Study the drawing (mm; zero at the part's minimum x, y, z) and answer. Give positions to 0.01 mm unless a question says otherwise; leave off trailing zeros. Write each loop counter-clockwise with the first axis right and the second up, starting at its lowest first coordinate (ties: lowest second). Pieces come first, ordered by that corner, then holes.
1) Find section A-A (y = 112). Determine the outline of the cut face in (x, z), plus the area to 3 significant figures.
2) Given pin 1 Ø3 at (y, z) = (112, 5) entering from -X; pin 2 Ø8 at (y, z) = (132, 24.5) entering from +X; pin 3 Ø3 at (x, z) = (38.5, 30) entering from -Y, each flat-ended and moving along its own axis, determine where each tip first touches the part or whether it passes through.
3) Straight lines are drawn through the part: probe 1 along Y at (x, z) = (64, 7); probe 2 along Y at (x, z) = (119.5, 21); probe 3 along X at (y, z) = (32.5, 28). For each, find the intervals that lie inside material, in ascending order.
4) Find section C-C (x = 67). Determine the outline of the cut face in (y, z), plus the area to 3 significant figures.
5) Find section B-B (z = 13). Determine the outline of the cut face in (x, y).
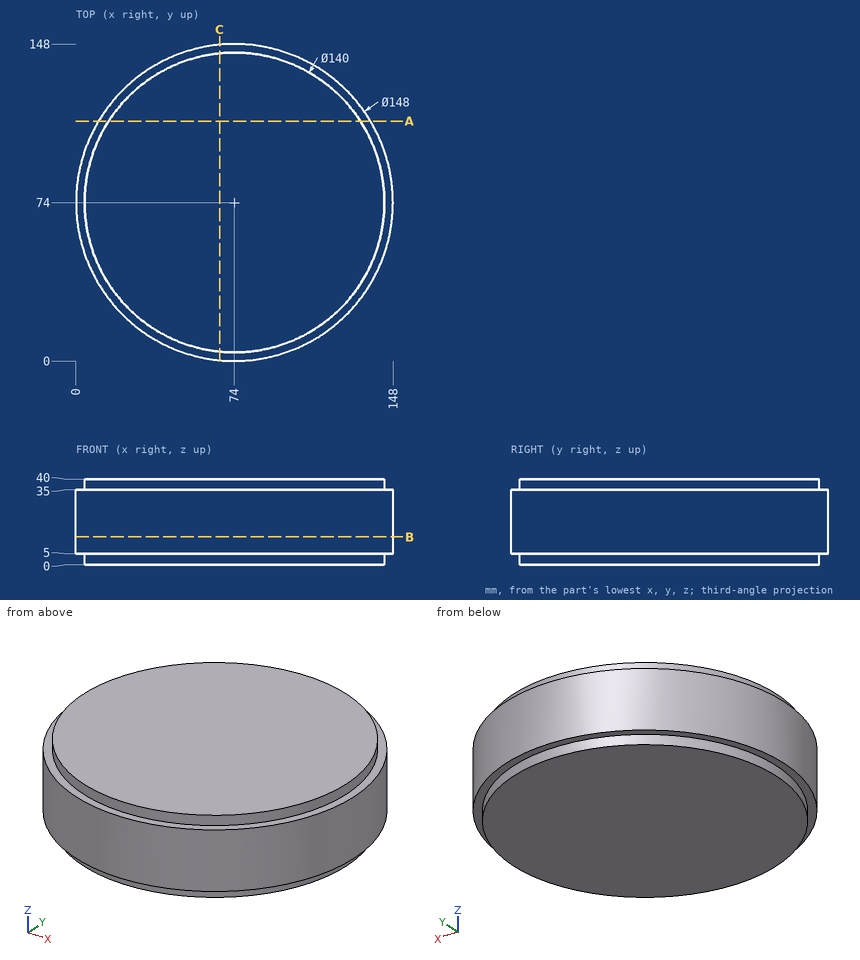
Results:
1. outline: (10.5, 5) - (15.21, 5) - (15.21, 0) - (132.79, 0) - (132.79, 5) - (137.5, 5) - (137.5, 35) - (132.79, 35) - (132.79, 40) - (15.21, 40) - (15.21, 35) - (10.5, 35) - close
1. area: 4,990 mm2
2. pin 1: stops at x = 9.63
2. pin 2: stops at x = 124.6
2. pin 3: stops at y = 8.27
3. probe 1: y = 0.68 to 147.32
3. probe 2: y = 15.64 to 132.36
3. probe 3: x = 12.73 to 135.27
4. outline: (0.33, 5) - (4.35, 5) - (4.35, 0) - (143.65, 0) - (143.65, 5) - (147.67, 5) - (147.67, 35) - (143.65, 35) - (143.65, 40) - (4.35, 40) - (4.35, 35) - (0.33, 35) - close
4. area: 5,810 mm2
5. outline: circle Ø148 at (74, 74)
